The listing builds one solid part. Answer for the finished solid, in the listing's coordinates (mm). Give positions to 0.01 mm unless a question says otherwise; leave off trailing zeros. Write each loop counter-clockwise with the first axis right and the second up, starting at its lowest first coordinate (ties: lowest second). Pieces come first, ordered by that corner, then holes.
```python
from build123d import *

# Parameters (mm, degrees)
SKETCH1_R           = 2.9337
BOSS_EXTRUDE1_DEPTH = 101.6


with BuildPart() as part:
    # Sketch1 → Boss-Extrude1 (new body)
    with BuildSketch(Plane.XY):
        with BuildLine():
            Line((-1.587500385, 6.349999904), (-3.666174594, 6.349999778))
            Line((-3.666174594, 6.349999778), (-4.70551159, 4.549815043))
            ThreePointArc((-4.70551159, 4.549815043), (-4.12444613, 2.38124975), (-6.293011423, 1.80018429))
            Line((-6.293011423, 1.80018429), (-7.332348419, -4.44e-07))
            Line((-7.332348419, -4.44e-07), (-6.293011205, -1.800185053))
            ThreePointArc((-6.293011205, -1.800185053), (-4.124445841, -2.38125025), (-4.705511038, -4.549815614))
            Line((-4.705511038, -4.549815614), (-3.666173825, -6.350000222))
            Line((-3.666173825, -6.350000222), (-1.587499615, -6.350000096))
            ThreePointArc((-1.587499615, -6.350000096), (2.89e-07, -4.7625), (1.587500385, -6.349999904))
            Line((1.587500385, -6.349999904), (3.666174594, -6.349999778))
            Line((3.666174594, -6.349999778), (4.70551159, -4.549815043))
            ThreePointArc((4.70551159, -4.549815043), (4.12444613, -2.38124975), (6.293011423, -1.80018429))
            Line((6.293011423, -1.80018429), (7.332348419, 4.44e-07))
            Line((7.332348419, 4.44e-07), (6.293011205, 1.800185053))
            ThreePointArc((6.293011205, 1.800185053), (4.124445841, 2.38125025), (4.705511038, 4.549815614))
            Line((4.705511038, 4.549815614), (3.666173825, 6.350000222))
            Line((3.666173825, 6.350000222), (1.587499615, 6.350000096))
            ThreePointArc((1.587499615, 6.350000096), (-2.89e-07, 4.7625), (-1.587500385, 6.349999904))
        make_face()
        Circle(SKETCH1_R, mode=Mode.SUBTRACT)
    extrude(amount=BOSS_EXTRUDE1_DEPTH)


solid = part.part
```
Item 1: Consider probe 1 along Y at (x, z) = (0, 60); probe 2 along Y at (x, z) = (1.25, 20); probe 3 along X at (y, z) = (-2.25, 54). Determine where each line is inside the solid, lowest interval first.
Conclusion:
probe 1: y = -4.76 to -2.93, 2.93 to 4.76
probe 2: y = -5.37 to -2.65, 2.65 to 5.37
probe 3: x = -4.21 to -1.88, 1.88 to 4.21
Item 2: Each of these flat-tipped pins is pushed along its axis until it touches: P1, Ø6, axis at x = -3.5, y = -2.5, coming from the -Z side; P2, Ø2, axis at y = -4, z = 63, coming from the +X side; P3, Ø2, axis at y = 4.5, z = 50.5, coming from the -X side; P4, Ø4, axis at y = -3, z = 67, coming from the -X side (3 decimals). Where does it stop, or does it pass through?
Conclusion:
P1: stops at z = 0
P2: stops at x = 4.71
P3: stops at x = -4.71
P4: stops at x = -6.755
Item 3: A cutting plane is placed at A-A, the plane x = 0. Give the vertices of the cut face in (y, z), plus the area to 3 significant figures.
Conclusion:
outline: (-4.76, 0) - (-2.93, 0) - (-2.93, 101.6) - (-4.76, 101.6) - close; (2.93, 0) - (4.76, 0) - (4.76, 101.6) - (2.93, 101.6) - close
area: 372 mm2
